CAD build for the part. Positions are in the model's coordinates, mm. A direction names the side the tool comes from. Round coordinates to 2 decimals unless told otherwise and drop trailing zeros. Order: outer loops, then holes, each group sorted by start corner. A loop starts at its lowest first (then second) coordinate and runs counter-clockwise, first axis right, second up. Notation, with made-up numbers: (-21, 69) - (32, 69) arc R24 ccw to (32, 84) - close; hole circle Ø9 at (83, 37). An arc over 180 degrees is marked (long way). Use one line per item in the form item = value. Start each with the question number.
from build123d import *

# Parameters (mm, degrees)
SKETCH1_W           = 38
SKETCH1_H           = 32.2
SKETCH1_R           = 2.625
BOSS_EXTRUDE1_DEPTH = 3
SKETCH2_W           = 38
SKETCH2_H           = 3
BOSS_EXTRUDE2_DEPTH = 35
SKETCH3_R           = 2.625
CUT_EXTRUDE1_DEPTH  = 62.160771741
BOSS_EXTRUDE3_DEPTH = 38


with BuildPart() as part:
    # Sketch1 → Boss-Extrude1 (new body)
    with BuildSketch(Plane(origin=(0, 0, 0), x_dir=(1, 0, 0), z_dir=(0, 1, 0))):
        with Locations((-19, -16.1)):
            Rectangle(SKETCH1_W, SKETCH1_H)
        with Locations(Location((-29, -23.2, 0), (0, 0, 270))):
            Circle(SKETCH1_R, mode=Mode.SUBTRACT)
        with Locations(Location((-9, -23.2, 0), (0, 0, 90))):
            Circle(SKETCH1_R, mode=Mode.SUBTRACT)
    extrude(amount=BOSS_EXTRUDE1_DEPTH)

    # Sketch2 → Boss-Extrude2 (add)
    with BuildSketch(Plane(origin=(0, 3, 0), x_dir=(1, 0, 0), z_dir=(0, 1, 0))):
        with Locations((-19, -1.5)):
            Rectangle(SKETCH2_W, SKETCH2_H)
    extrude(amount=BOSS_EXTRUDE2_DEPTH)

    # Sketch3 → Cut-Extrude1 (cut, through all)
    with BuildSketch(Plane.XY.offset(3)):
        with Locations((-29, 25)):
            Circle(SKETCH3_R)
        with Locations((-9, 25)):
            Circle(SKETCH3_R)
    extrude(amount=-CUT_EXTRUDE1_DEPTH, mode=Mode.SUBTRACT)

    # Sketch4 → Boss-Extrude3 (add, through all)
    with BuildSketch(Plane(origin=(0, 0, 0), x_dir=(0, 0, -1), z_dir=(1, 0, 0))):
        Polygon((-3, 8), (-8, 3), (-3, 3), align=None)
    extrude(amount=-BOSS_EXTRUDE3_DEPTH)


solid = part.part
(1) Flat gauge pins, fed straight in: P1, Ø15, axis at x = -23.5, y = 21, coming from the +Z side; P2, Ø6, axis at x = -16, z = 13.5, coming from the -Y side. Where does each tip first touch, or does it go through?
(2) Slice it at A-A (x = -9). Give the cut face in (y, z) (3 decimals), and give its area (3 significant figures).
(3) Slice it at B-B (z = 23.2). Give the cut face in (x, y) (3 decimals).
(4) Which spindle directions (+Z, -Z, +X, -X, +Y, -Y) get a long thin tool onto all of the face, cutting with end or side? Do faces 5 (the flat face through (-19, 19, 0)), 6 (the flat face through (-19, 3, 20)). Say none if no direction does.
(5) Wall check: line 1 (X direction, y = 1.55, z = 23.2) (3 decimals); line 2 (Z direction, x = -9, y = 1) (3 decimals); line 3 (Y direction, x = -9, z = 2.15) (3 decimals). Give the ranges that are in metal, low to high. Write a range as [from, to].
(6) Mould opens along X. For faces 1 (the cylindrical face through (-9.115, 1.479, 25.822)), 2 (the cylindrical face through (-31.563, 1.479, 22.631)), 3 (the flat face through (-19, 23, 3)), 4 (the flat face through (0, 6, 4)) say: pulls with the +X half, pulls with the -X half, needs draft (parallel to the pull), parting line crosses it, or undercut.
(7) Slice it at D-D (x = -35). Give the cut face in (y, z), and give its area (3 significant figures).
Results list:
q1.P1 = 3
q1.P2 = 0
q2.outline = (0, 0) - (22.375, 0) - (22.375, 3) - (8, 3) - (3, 8) - (3, 20.575) - (0, 20.575) - close; (0, 25.825) - (3, 25.825) - (3, 32.2) - (0, 32.2) - close; (27.625, 0) - (38, 0) - (38, 3) - (27.625, 3) - close
q2.area = 183 mm²
q3.outline = (-38, 0) - (-31.625, 0) - (-31.625, 3) - (-38, 3) - close; (-26.375, 0) - (-11.625, 0) - (-11.625, 3) - (-26.375, 3) - close; (-6.375, 0) - (0, 0) - (0, 3) - (-6.375, 3) - close
q4.face_5 = -Z, +X, -X, +Y, -Y
q4.face_6 = +Z, +X, -X, +Y
q5.line_1 = [-38, -31.625], [-26.375, -11.625], [-6.375, 0]
q5.line_2 = [0, 20.575], [25.825, 32.2]
q5.line_3 = [0, 22.375], [27.625, 38]
q6.face_1 = undercut
q6.face_2 = undercut
q6.face_3 = needs draft
q6.face_4 = pulls with the +X half
q7.outline = (0, 0) - (38, 0) - (38, 3) - (8, 3) - (3, 8) - (3, 32.2) - (0, 32.2) - close
q7.area = 214 mm²
